Could you check a few things on this model? Use its own coordinates, in mm. A direction names the side the tool comes from. Round coordinates to 2 decimals unless told otherwise and drop trailing zeros. Order: outer loops, then holes, each group sorted by start corner. A loop starts at its lowest first (then second) coordinate and runs counter-clockwise, first axis right, second up. Notation, with made-up numbers: (22, 87) -> (69, 87) arc R25 cw to (69, 118) -> close; hole circle Ø9 at (33.25, 88.25). An arc over 180 degrees is marked (long way). One line per question, with ' | ' between items.
```python
from build123d import *

# Parameters (mm, degrees)
EXTRUDE_1_DEPTH          = 7.5
CUT_EXTRUDE_1_DEPTH      = 30.546573405
CUT_EXTRUDE_1_DEPTH_BACK = 30.546573405
SKETCH_2_W               = 20
SKETCH_2_H               = 20
FILLET_1_R               = 5
FILLET_2_R               = 5
CUT_EXTRUDE_2_DEPTH      = 41.942032192
CUT_EXTRUDE_2_DEPTH_BACK = 41.942032192
SKETCH_3_R               = 4.1
CUT_EXTRUDE_3_DEPTH      = 41.942032192
CUT_EXTRUDE_3_DEPTH_BACK = 41.942032192
SKETCH_4_R               = 4.1
EXTRUDE_START            = 20
EXTRUDE_2_DEPTH          = 20
EXTRUDE_START_2          = -4
SKETCH_6_R               = 4.1
SKETCH_6_R_2             = 3.5
EXTRUDE_3_DEPTH          = 4
SKETCH_7_R               = 4.1
SKETCH_7_R_2             = 3.5
EXTRUDE_4_DEPTH          = 4
EXTRUDE_START_3          = -8
SKETCH_8_R               = 4.1
SKETCH_8_R_2             = 3.5
EXTRUDE_5_DEPTH          = 4
SKETCH_9_R               = 4.1
SKETCH_9_R_2             = 3.5
EXTRUDE_6_DEPTH          = 4


with BuildPart() as part:
    # ｽｹｯﾁ1 → ﾎﾞｽ - 押し出し1 (new, symmetric)
    with BuildSketch(Plane.XY):
        Polygon((7.455844123, -18), (18, -7.455844123), (18, 7.455844123), (7.455844123, 18), (-7.455844123, 18), (-18, 7.455844123), (-18, -7.455844123), (-7.455844123, -18), align=None)
    extrude(amount=EXTRUDE_1_DEPTH, both=True)

    # ｽｹｯﾁ2 → ｶｯﾄ - 押し出し1 (cut, two sides: drawn at the far end of the back side and taken through both)
    with BuildSketch(Plane.XY.offset(7.5).offset(-CUT_EXTRUDE_1_DEPTH_BACK)):
        Rectangle(SKETCH_2_W, SKETCH_2_H)
    extrude(amount=CUT_EXTRUDE_1_DEPTH + CUT_EXTRUDE_1_DEPTH_BACK, mode=Mode.SUBTRACT)

    # ﾌｨﾚｯﾄ1
    fillet_1_edges = [part.edges().sort_by_distance(p)[0] for p in [
        (-10, -10, 0),
        (-10, 10, 0),
        (10, 10, 0),
        (10, -10, 0),
    ]]
    fillet(fillet_1_edges, radius=FILLET_1_R)

    # ﾌｨﾚｯﾄ2
    fillet_2_edges = [part.edges().sort_by_distance(p)[0] for p in [
        (-7.455844123, 18, 0),
        (7.455844123, 18, 0),
        (18, 7.455844123, 0),
        (18, -7.455844123, 0),
        (7.455844123, -18, 0),
        (-7.455844123, -18, 0),
        (-18, -7.455844123, 0),
        (-18, 7.455844123, 0),
    ]]
    fillet(fillet_2_edges, radius=FILLET_2_R)

    # ｽｹｯﾁ3 → ｶｯﾄ - 押し出し2 (cut, two sides: drawn at the far end of the back side and taken through both)
    with BuildSketch(Plane.XZ.offset(18).offset(-CUT_EXTRUDE_2_DEPTH_BACK)):
        with Locations(Location((0, 0, 0), (0, 0, 270))):
            Circle(SKETCH_3_R)
    extrude(amount=CUT_EXTRUDE_2_DEPTH + CUT_EXTRUDE_2_DEPTH_BACK, mode=Mode.SUBTRACT)

    # ｽｹｯﾁ4 → ｶｯﾄ - 押し出し3 (cut, two sides: drawn at the far end of the back side and taken through both)
    with BuildSketch(Plane(origin=(18, 0, 0), x_dir=(0, 0, -1), z_dir=(1, 0, 0)).offset(-CUT_EXTRUDE_3_DEPTH_BACK)):
        Circle(SKETCH_4_R)
    extrude(amount=CUT_EXTRUDE_3_DEPTH + CUT_EXTRUDE_3_DEPTH_BACK, mode=Mode.SUBTRACT)

    # ｽｹｯﾁ5 → ﾎﾞｽ - 押し出し2 (add)
    with BuildSketch(Plane.XY.offset(7.5).offset(EXTRUDE_START)):
        with BuildLine():
            Line((8.920310217, -16.535533906), (16.535533906, -8.920310217))
            ThreePointArc((16.535533906, -8.920310217), (17.619397663, -7.298193473), (18, -5.384776311))
            Line((18, -5.384776311), (18, 5.384776311))
            ThreePointArc((18, 5.384776311), (17.619397663, 7.298193473), (16.535533906, 8.920310217))
            Line((16.535533906, 8.920310217), (8.920310217, 16.535533906))
            ThreePointArc((8.920310217, 16.535533906), (7.298193473, 17.619397663), (5.384776311, 18))
            Line((5.384776311, 18), (-5.384776311, 18))
            ThreePointArc((-5.384776311, 18), (-7.298193473, 17.619397663), (-8.920310217, 16.535533906))
            Line((-8.920310217, 16.535533906), (-16.535533906, 8.920310217))
            ThreePointArc((-16.535533906, 8.920310217), (-17.619397663, 7.298193473), (-18, 5.384776311))
            Line((-18, 5.384776311), (-18, -5.384776311))
            ThreePointArc((-18, -5.384776311), (-17.619397663, -7.298193473), (-16.535533906, -8.920310217))
            Line((-16.535533906, -8.920310217), (-8.920310217, -16.535533906))
            ThreePointArc((-8.920310217, -16.535533906), (-7.298193473, -17.619397663), (-5.384776311, -18))
            Line((-5.384776311, -18), (5.384776311, -18))
            ThreePointArc((5.384776311, -18), (7.298193473, -17.619397663), (8.920310217, -16.535533906))
        make_face()
        with BuildLine():
            Line((5, 10), (-5, 10))
            ThreePointArc((-5, 10), (-8.535533906, 8.535533906), (-10, 5))
            Line((-10, 5), (-10, -5))
            ThreePointArc((-10, -5), (-8.535533906, -8.535533906), (-5, -10))
            Line((-5, -10), (5, -10))
            ThreePointArc((5, -10), (8.535533906, -8.535533906), (10, -5))
            Line((10, -5), (10, 5))
            ThreePointArc((10, 5), (8.535533906, 8.535533906), (5, 10))
        make_face(mode=Mode.SUBTRACT)
    extrude(amount=-EXTRUDE_2_DEPTH)

    # ｽｹｯﾁ6 → ﾎﾞｽ - 押し出し3 (add)
    with BuildSketch(Plane.XZ.offset(18).offset(EXTRUDE_START_2)):
        Circle(SKETCH_6_R)
        Circle(SKETCH_6_R_2, mode=Mode.SUBTRACT)
    extrude(amount=-EXTRUDE_3_DEPTH)

    # ｽｹｯﾁ7 → ﾎﾞｽ - 押し出し4 (add)
    with BuildSketch(Plane(origin=(18, 0, 0), x_dir=(0, 0, -1), z_dir=(1, 0, 0)).offset(EXTRUDE_START_2)):
        with Locations(Location((0, 0, 0), (0, 0, 90))):
            Circle(SKETCH_7_R)
        Circle(SKETCH_7_R_2, mode=Mode.SUBTRACT)
    extrude(amount=-EXTRUDE_4_DEPTH)

    # ｽｹｯﾁ8 → ﾎﾞｽ - 押し出し5 (add)
    with BuildSketch(Plane(origin=(0, 18, 0), x_dir=(1, 0, 0), z_dir=(0, 1, 0)).offset(EXTRUDE_START_3)):
        Circle(SKETCH_8_R)
        Circle(SKETCH_8_R_2, mode=Mode.SUBTRACT)
    extrude(amount=EXTRUDE_5_DEPTH)

    # ｽｹｯﾁ9 → ﾎﾞｽ - 押し出し6 (add)
    with BuildSketch(Plane.ZY.offset(18).offset(EXTRUDE_START_3)):
        with Locations(Location((0, 0, 0), (0, 0, 90))):
            Circle(SKETCH_9_R)
        with Locations(Location((0, 0, 0), (0, 0, 180))):
            Circle(SKETCH_9_R_2, mode=Mode.SUBTRACT)
    extrude(amount=EXTRUDE_6_DEPTH)


solid = part.part
```
1. I want a section at A-A on x = 0. List the corners of the cut face in (y, z) for me, and give its area (3 significant figures).
From the geometry:
outline: (-18, -7.5) -> (-10, -7.5) -> (-10, -3.5) -> (-14, -3.5) -> (-14, -4.1) -> (-18, -4.1) -> close; (-18, 4.1) -> (-14, 4.1) -> (-14, 3.5) -> (-10, 3.5) -> (-10, 27.5) -> (-18, 27.5) -> close; (10, -7.5) -> (18, -7.5) -> (18, -4.1) -> (14, -4.1) -> (14, -3.5) -> (10, -3.5) -> close; (10, 3.5) -> (14, 3.5) -> (14, 4.1) -> (18, 4.1) -> (18, 27.5) -> (10, 27.5) -> close | area: 438 mm²
2. On a 3-axis mill with a long thin cutter (end or side, diameter ignored), from which of +Z, -Z, +X, -X, +Y, -Y can I reach the whole of each face in a straight line? I mean faces 4 (the face through (-16.03, 1.23, -3.91)), 5 (the face through (15.97, 1.23, -3.91)), 6 (the face through (0, 10, 10)). Say none if no direction works.
From the geometry:
face 4: -X | face 5: +X | face 6: +Z, -Z
3. I'm going to push flat-ended pins straight in: pin 1 (8 mm diameter, centred on x = -11, z = 1, fed in from +Y); pin 2 (12 mm diameter, centred on y = 12.5, z = 22, fed in from -X); pin 3 (8 mm diameter, centred on y = -1, z = 3, fed in from +X); pin 4 (4 mm diameter, centred on x = -8, z = 18.5, fed in from -Y). Where does each tip first touch, or does it pass through?
From the geometry:
pin 1: stops at y = 17.73 | pin 2: stops at x = -17.87 | pin 3: stops at x = 18 | pin 4: stops at y = -17.96
4. I need wall thicknesses on probe 1 along X at (y, z) = (-1, 21); probe 2 along Z at (x, y) = (-16.65, 0); probe 3 along Y at (x, z) = (-15.65, 0). Which ranges of each line are inside material? Lowest first, please.
From the geometry:
probe 1: x = -18 to -10, 10 to 18 | probe 2: z = -7.5 to -4.1, 4.1 to 27.5 | probe 3: y = -9.81 to -4.1, 4.1 to 9.81
5. I want a section at D-D on y = -13.5. List the corners of the cut face in (x, z) for me.
From the geometry:
outline: (-11.96, -7.5) -> (11.96, -7.5) -> (11.96, 27.5) -> (-11.96, 27.5) -> close; hole circle Ø7 at (0, 0)
6. I want a section at C-C on x = -7. List the corners of the cut face in (y, z) for me.
From the geometry:
outline: (-17.73, -7.5) -> (-9.58, -7.5) -> (-9.58, 27.5) -> (-17.73, 27.5) -> close; (9.58, -7.5) -> (17.73, -7.5) -> (17.73, 27.5) -> (9.58, 27.5) -> close
7. If we mould it in two halves opening along X, with no side actions, what happens to faces 1 (the face through (12.675, -12.781, 10.245)), 2 (the face through (10, 0, 10)), 3 (the face through (-12.675, 12.781, 10.245))? For each: pulls with the +X half, pulls with the -X half, needs draft (parallel to the pull), parting line crosses it, or undercut.
From the geometry:
face 1: pulls with the +X half | face 2: undercut | face 3: pulls with the -X half
